from build123d import *

# Parameters (mm, degrees)
SKETCH1_W           = 20
SKETCH1_H           = 11
SKETCH1_W_2         = 7
SKETCH1_H_2         = 5
SKETCH1_R           = 3.25
SKETCH1_R_2         = 1.5
SKETCH1_W_3         = 8
BOSS_EXTRUDE1_DEPTH = 1
SKETCH1_3_W         = 7
SKETCH1_3_H         = 5
BOSS_EXTRUDE2_DEPTH = 7
BOSS_EXTRUDE3_START = 1
SKETCH1_4_W         = 8
SKETCH1_4_H         = 11
BOSS_EXTRUDE3_DEPTH = 6
SKETCH3_W           = 8
SKETCH3_H           = 5
BOSS_EXTRUDE4_DEPTH = 2
SKETCH4_R           = 0.75
BOSS_EXTRUDE6_DEPTH = 3


with BuildPart() as part:
    # Sketch1 → Boss-Extrude1 (new body)
    # profile 1 of 4: a face of its own
    with BuildSketch(Plane(origin=(0, 0, 0), x_dir=(1, 0, 0), z_dir=(0, 1, 0))):
        with Locations((-4, 0)):
            Rectangle(SKETCH1_W, SKETCH1_H)
        with Locations((-9.5, 0)):
            Rectangle(SKETCH1_W_2, SKETCH1_H_2, mode=Mode.SUBTRACT)
        Circle(SKETCH1_R, mode=Mode.SUBTRACT)
    # profile 2 of 4: a face of its own
    with BuildSketch(Plane(origin=(0, 0, 0), x_dir=(1, 0, 0), z_dir=(0, 1, 0))):
        with Locations((-9.5, 0)):
            Rectangle(SKETCH1_W_2, SKETCH1_H_2)
    # profile 3 of 4: a face of its own
    with BuildSketch(Plane(origin=(0, 0, 0), x_dir=(1, 0, 0), z_dir=(0, 1, 0))):
        Circle(SKETCH1_R)
        with Locations(Location((0, 0, 0), (0, 0, 270))):
            Circle(SKETCH1_R_2, mode=Mode.SUBTRACT)
    # profile 4 of 4: a face of its own
    with BuildSketch(Plane(origin=(0, 0, 0), x_dir=(1, 0, 0), z_dir=(0, 1, 0))):
        with Locations((10, 0)):
            Rectangle(SKETCH1_W_3, SKETCH1_H)
    extrude(amount=BOSS_EXTRUDE1_DEPTH)

    # Sketch1<3> → Boss-Extrude2 (add)
    with BuildSketch(Plane(origin=(0, 0, 0), x_dir=(1, 0, 0), z_dir=(0, 1, 0))):
        with Locations((-9.5, 0)):
            Rectangle(SKETCH1_3_W, SKETCH1_3_H)
    extrude(amount=-BOSS_EXTRUDE2_DEPTH)

    # Sketch1<4> → Boss-Extrude3 (add)
    with BuildSketch(Plane(origin=(0, 0, 0), x_dir=(1, 0, 0), z_dir=(0, 1, 0)).offset(BOSS_EXTRUDE3_START)):
        with Locations((10, 0)):
            Rectangle(SKETCH1_4_W, SKETCH1_4_H)
    extrude(amount=BOSS_EXTRUDE3_DEPTH)

    # Sketch3 → Boss-Extrude4 (add)
    with BuildSketch(Plane(origin=(14, 0, 0), x_dir=(0, 0, -1), z_dir=(1, 0, 0))):
        with Locations((0, 3.5)):
            Rectangle(SKETCH3_W, SKETCH3_H)
    extrude(amount=BOSS_EXTRUDE4_DEPTH)

    # Sketch4 → Boss-Extrude6 (add)
    with BuildSketch(Plane(origin=(16, 0, 0), x_dir=(0, 0, -1), z_dir=(1, 0, 0))):
        with Locations(Location((-2, 3.603838689, 0), (0, 0, 180))):
            Circle(SKETCH4_R)
        with Locations(Location((0, 3.603838689, 0), (0, 0, 180))):
            Circle(SKETCH4_R)
        with Locations(Location((2, 3.603838689, 0), (0, 0, 180))):
            Circle(SKETCH4_R)
    extrude(amount=BOSS_EXTRUDE6_DEPTH)


solid = part.part
Verification items for the finished model (mm, model axes). A direction names the side the tool comes from. Round coordinates to 2 decimals unless told otherwise and drop trailing zeros. Loops run counter-clockwise (first coordinate to the right, second up) from the corner with the lowest first, then second, coordinate; pieces in that order, holes last. Notation, with made-up numbers: (44.5, 51.25) - (65.5, 51.25) arc R18 cw to (65.5, 82.25) - close; hole circle Ø3 at (15.25, -17.75). An arc over 180 degrees is marked (long way). Write item = value, one per line.
Q1. Material ranges on L1, parallel to X at y = 0.45, z = 0; L2, parallel to Y at x = 12.5, z = -1.75; L3, parallel to Z at x = -11.5, y = -1.5, recorded low to high.
Here are the results:
L1 = -14 to -1.5, 1.5 to 14
L2 = 0 to 7
L3 = -2.5 to 2.5
Q2. Mould release check, pull along Z, two halves, no side actions. Record for faces 1 (the flat face through (15, 3, 4)), 2 (the flat face through (6, 4, 0)), 3 (the flat face through (15, 3, -4)), 4 (the cylindrical face through (17.48, 2.97, 0.4)): +Z half, -Z half, draft (parallel to the pull), parting line (faces both ways), or undercut.
Here are the results:
face_1 = +Z half
face_2 = draft
face_3 = -Z half
face_4 = undercut
Q3. Depth check by flat-ended pin: pin 1 (3.5 mm diameter, centred on x = -9, y = -4, fed in from +Z); pin 2 (4 mm diameter, centred on x = 0, z = 0, fed in from +Y); pin 3 (1.5 mm diameter, centred on y = -4, z = -0.5, fed in from +X). Enter the tip coordinate at first touch or a pass-through.
Here are the results:
pin_1 = 2.5
pin_2 = 1
pin_3 = -6
Q4. Sectioned sample at B-B on z = 0. Record the boundary of the cut face in (x, y).
Here are the results:
outline = (-14, 0) - (-13, 0) - (-13, -7) - (-6, -7) - (-6, 0) - (-1.5, 0) - (-1.5, 1) - (-14, 1) - close; (1.5, 0) - (14, 0) - (14, 1) - (16, 1) - (16, 2.85) - (19, 2.85) - (19, 4.35) - (16, 4.35) - (16, 6) - (14, 6) - (14, 7) - (6, 7) - (6, 1) - (1.5, 1) - close
Q5. Sectioned sample at C-C on z = -2. Record the boundary of the cut face in (x, y).
Here are the results:
outline = (-14, 0) - (-13, 0) - (-13, -7) - (-6, -7) - (-6, 0) - (14, 0) - (14, 1) - (16, 1) - (16, 2.85) - (19, 2.85) - (19, 4.35) - (16, 4.35) - (16, 6) - (14, 6) - (14, 7) - (6, 7) - (6, 1) - (-14, 1) - close
Q6. Tool access check on faces 5 (the flat face through (-4, 1, 0)), 6 (the flat face through (15, 6, 0)), 7 (the flat face through (14, 6.6, 0.1)). Record the directions out of +Z, -Z, +X, -X, +Y, -Y that give a thin tool (end or side, any length) a straight path to the whole face; none if there is none.
Here are the results:
face_5 = +Z, -Z, -X, +Y
face_6 = +Z, -Z, +X, +Y
face_7 = +X
Q7. Sectioned sample at D-D on y = 1.5. Record the boundary of the cut face in (x, z).
Here are the results:
outline = (6, -5.5) - (14, -5.5) - (14, -4) - (16, -4) - (16, 4) - (14, 4) - (14, 5.5) - (6, 5.5) - close
Q8. Sectioned sample at A-A on x = 0. Record the boundary of the cut face in (y, z).
Here are the results:
outline = (0, -5.5) - (1, -5.5) - (1, -1.5) - (0, -1.5) - close; (0, 1.5) - (1, 1.5) - (1, 5.5) - (0, 5.5) - close
